from build123d import *

# Parameters (mm, degrees)
SKETCH1_R           = 50
BOSS_EXTRUDE1_DEPTH = 5
FILLET1_R           = 5
SKETCH2_R           = 1.9
CUT_EXTRUDE1_DEPTH  = 5


with BuildPart() as part:
    # Sketch1 → Boss-Extrude1 (new body)
    with BuildSketch(Plane.XY):
        Circle(SKETCH1_R)
        with BuildLine():
            Line((30.504506916, 35.755769574), (0, 5.251262658))
            Line((0, 5.251262658), (-30.504506916, 35.755769574))
            ThreePointArc((-30.504506916, 35.755769574), (0, 47), (30.504506916, 35.755769574))
        make_face(mode=Mode.SUBTRACT)
        with BuildLine():
            Line((5.251262658, 0), (35.755769574, 30.504506916))
            ThreePointArc((35.755769574, 30.504506916), (47, 0), (35.755769574, -30.504506916))
            Line((35.755769574, -30.504506916), (5.251262658, 0))
        make_face(mode=Mode.SUBTRACT)
        with BuildLine():
            Line((0, -5.251262658), (30.504506916, -35.755769574))
            ThreePointArc((30.504506916, -35.755769574), (0, -47), (-30.504506916, -35.755769574))
            Line((-30.504506916, -35.755769574), (0, -5.251262658))
        make_face(mode=Mode.SUBTRACT)
        with BuildLine():
            Line((-5.251262658, 0), (-35.755769574, -30.504506916))
            ThreePointArc((-35.755769574, -30.504506916), (-47, 0), (-35.755769574, 30.504506916))
            Line((-35.755769574, 30.504506916), (-5.251262658, 0))
        make_face(mode=Mode.SUBTRACT)
    extrude(amount=BOSS_EXTRUDE1_DEPTH)

    # Fillet1
    fillet1_edges = [part.edges().sort_by_distance(p)[0] for p in [
        (-5.251262658, 0, 2.5),
        (-35.755769574, 30.504506916, 2.5),
        (-35.755769574, -30.504506916, 2.5),
        (35.755769574, -30.504506916, 2.5),
        (35.755769574, 30.504506916, 2.5),
        (5.251262658, 0, 2.5),
        (-30.504506916, -35.755769574, 2.5),
        (30.504506916, -35.755769574, 2.5),
        (0, -5.251262658, 2.5),
        (30.504506916, 35.755769574, 2.5),
        (-30.504506916, 35.755769574, 2.5),
        (0, 5.251262658, 2.5),
    ]]
    fillet(fillet1_edges, radius=FILLET1_R)

    # Sketch2 → Cut-Extrude1 (cut)
    with BuildSketch(Plane.XY.offset(5)):
        with Locations((5.656854249, -5.656854249)):
            Circle(SKETCH2_R)
        with Locations((5.656854249, 5.656854249)):
            Circle(SKETCH2_R)
        with Locations((-5.656854249, 5.656854249)):
            Circle(SKETCH2_R)
        with Locations((-5.656854249, -5.656854249)):
            Circle(SKETCH2_R)
    extrude(amount=-CUT_EXTRUDE1_DEPTH, mode=Mode.SUBTRACT)


solid = part.part
Work out the finished part from the listing and answer in its coordinate system (mm). Round coordinates to 2 decimals unless told otherwise and drop trailing zeros. Loops run counter-clockwise (first coordinate to the right, second up) from the corner with the lowest first, then second, coordinate; pieces in that order, holes last. Notation, with made-up numbers: (0.5, -4) - (10.5, -4) arc R22 cw to (10.5, 17) - close; hole circle Ø3 at (56.5, 16.25). An arc over 180 degrees is marked (long way). Use one line per item in the form item = value. Start each with the question number.
(1) Determine the mould class of faces 1 (the face through (5.41, 7.54, 2.54)), 2 (the face through (0, 0, 5)) for opening direction Y: +Y half, -Y half, draft (parallel to the pull), parting line (faces both ways), or undercut.
(2) Find section C-C on x = -18. Determine the outline of the cut face in (y, z), and give its area (3 significant figures).
(3) Consider line 1 (Y direction, x = 24.5, z = 2.15); line 2 (X direction, y = -6, z = 1.3); line 3 (Y direction, x = -10.5, z = 1.3). Determine where each line is inside the solid, lowest interval first.
(4) Find section A-A on x = 0. Determine the outline of the cut face in (y, z).
(5) Flat-ended cylindrical pins translate along their axes: P1, Ø3, axis at y = -17, z = 4.5, coming from the -X side; P2, Ø3, axis at y = -37.5, z = 2, coming from the +X side; P3, Ø1.5, axis at y = -3, z = 3, coming from the +X side. Find the tip coordinate at first contact, or state that the pin passes through.
(6) Find section B-B on y = -17.5. Determine the outline of the cut face in (x, z), and give its area (3 significant figures).
Answer list:
q1.face_1 = undercut
q1.face_2 = draft
q2.outline = (-46.65, 0) - (-43.42, 0) - (-43.42, 5) - (-46.65, 5) - close; (-23.25, 0) - (-12.75, 0) - (-12.75, 5) - (-23.25, 5) - close; (12.75, 0) - (23.25, 0) - (23.25, 5) - (12.75, 5) - close; (43.42, 0) - (46.65, 0) - (46.65, 5) - (43.42, 5) - close
q2.area = 137 mm^2
q3.line_1 = -43.59 to -40.11, -29.75 to -19.25, 19.25 to 29.75, 40.11 to 43.59
q3.line_2 = -49.64 to -46.62, -11.25 to -7.53, -3.79 to 3.79, 7.53 to 11.25, 46.62 to 49.64
q3.line_3 = -48.89 to -45.81, -15.75 to -5.25, 5.25 to 15.75, 45.81 to 48.89
q4.outline = (-50, 0) - (-47, 0) - (-47, 5) - (-50, 5) - close; (-7.32, 0) - (7.32, 0) - (7.32, 5) - (-7.32, 5) - close; (47, 0) - (50, 0) - (50, 5) - (47, 5) - close
q5.P1 = -47.54
q5.P2 = 34.7
q5.P3 = 49.95
q6.outline = (-46.84, 0) - (-43.62, 0) - (-43.62, 5) - (-46.84, 5) - close; (-22.75, 0) - (-12.25, 0) - (-12.25, 5) - (-22.75, 5) - close; (12.25, 0) - (22.75, 0) - (22.75, 5) - (12.25, 5) - close; (43.62, 0) - (46.84, 0) - (46.84, 5) - (43.62, 5) - close
q6.area = 137 mm^2
